Verification items for the finished model (mm, model axes). A direction names the side the tool comes from. Give positions to 0.01 mm unless a question says otherwise; leave off trailing zeros. Loops run counter-clockwise (first coordinate to the right, second up) from the corner with the lowest first, then second, coordinate; pieces in that order, holes last. Notation, with made-up numbers: M 34.5,-26 L 38.5,-26 A18 cw 38.5,2 Z; hole C 77,-32 d4. An arc over 180 degrees is marked long. Use a Markdown table: item, result.
from build123d import *

# Parameters (mm, degrees)
SKETCH_1_W                  = 130
SKETCH_1_H                  = 114
EXTRUDE_1_DEPTH             = 4
CHAMFER_1_SIZE              = 2.5
CHAMFER_1_SIZE2             = 4.330127019
FILLET_1_R                  = 5
FILLET_2_R                  = 3
FILLET_3_R                  = 3
SKETCH_2_R                  = 1.55
CUT_EXTRUDE_1_DEPTH         = 87.544786094
PATTERN_LINEAR_1_COUNT      = 2
PATTERN_LINEAR_1_PITCH      = 116
PATTERN_LINEAR_1_COUNT_DIR2 = 2
PATTERN_LINEAR_1_PITCH_DIR2 = 90
SKETCH_4_R                  = 2.9
CUT_EXTRUDE_2_DEPTH         = 1.8
PATTERN_LINEAR_2_COUNT      = 2
PATTERN_LINEAR_2_PITCH      = 116
PATTERN_LINEAR_2_COUNT_DIR2 = 2
PATTERN_LINEAR_2_PITCH_DIR2 = 90


with BuildPart() as part:
    # Эскиз1 → Бобышка-Вытянуть1 (new body)
    with BuildSketch(Plane(origin=(0, 0, 0), x_dir=(1, 0, 0), z_dir=(0, 1, 0))):
        Rectangle(SKETCH_1_W, SKETCH_1_H)
    extrude(amount=EXTRUDE_1_DEPTH)

    # Фаска1
    chamfer_1_edges = [part.edges().sort_by_distance(p)[0] for p in [
        (0, 4, 57),
    ]]
    chamfer_1_side = [part.faces().sort_by_distance(p)[0] for p in [
        (0, 2, 57),
    ]]
    chamfer(chamfer_1_edges, length=CHAMFER_1_SIZE, length2=CHAMFER_1_SIZE2, reference=chamfer_1_side[0])

    # Скругление1
    fillet_1_edges = [part.edges().sort_by_distance(p)[0] for p in [
        (0, 4, 52.669872981),
    ]]
    fillet(fillet_1_edges, radius=FILLET_1_R)

    # Скругление2
    # the kernel refuses this fillet: 3 mm, written as the material it takes off along each edge
    with BuildSketch(Plane(origin=(69.302949009, 1.5, 57), x_dir=(0, 0.4999999999999978, -0.8660254037844398), z_dir=(-1, 0, 0))) as fillet_2_piece_1:
        with BuildLine():
            CenterArc((1.721179604, 3), FILLET_2_R, 214.540406951, 55.459593049)
            Line((-0.75, 1.299038106), (-0.799423592, 1.265018868))
            ThreePointArc((-0.799423592, 1.265018868), (-0.426961524, 0.619519053), (-0.051961524, -0.03))
            Line((-0.051961524, -0.03), (0, -0.06))
            Line((0, -0.06), (1.721179604, -0.06))
            Line((1.721179604, -0.06), (1.721179604, 0))
        make_face()
    extrude(amount=138.605898019, mode=Mode.SUBTRACT)

    # Скругление3
    fillet_3_edges = [part.edges().sort_by_distance(p)[0] for p in [
        (-65, 2, -57),
        (65, 2, -57),
    ]]
    fillet(fillet_3_edges, radius=FILLET_3_R)

    # Эскиз2 → Вырез-Вытянуть1 (cut, through all)
    with BuildSketch(Plane(origin=(0, 4, 0), x_dir=(1, 0, 0), z_dir=(0, 1, 0))):
        with Locations(Location((-58, 50, 0), (0, 0, 270))):
            Circle(SKETCH_2_R)
    cut_extrude_1 = extrude(amount=-CUT_EXTRUDE_1_DEPTH, mode=Mode.SUBTRACT)

    # Линейный массив1: Cut-Extrude 1 2 × 2
    with Locations(*[(i * PATTERN_LINEAR_1_PITCH, 0, j * PATTERN_LINEAR_1_PITCH_DIR2) for i in range(PATTERN_LINEAR_1_COUNT) for j in range(PATTERN_LINEAR_1_COUNT_DIR2) if (i, j) != (0, 0)]):
        add(cut_extrude_1, mode=Mode.SUBTRACT)

    # Эскиз4 → Вырез-Вытянуть2 (cut)
    with BuildSketch(Plane(origin=(0, 4, 0), x_dir=(1, 0, 0), z_dir=(0, 1, 0))):
        with Locations(Location((-58, 50, 0), (0, 0, 270))):
            Circle(SKETCH_4_R)
    cut_extrude_2 = extrude(amount=-CUT_EXTRUDE_2_DEPTH, mode=Mode.SUBTRACT)

    # Линейный массив2: Cut-Extrude 2 2 × 2
    with Locations(*[(i * PATTERN_LINEAR_2_PITCH, 0, j * PATTERN_LINEAR_2_PITCH_DIR2) for i in range(PATTERN_LINEAR_2_COUNT) for j in range(PATTERN_LINEAR_2_COUNT_DIR2) if (i, j) != (0, 0)]):
        add(cut_extrude_2, mode=Mode.SUBTRACT)


solid = part.part
(1) Cross-section at B-B on z = 40. Record the cut outline in (x, y), then the cut area to 3 significant figures.
Results below:
| item | result |
|---|---|
| outline | M -65,0 L -59.55,0 L -59.55,2.2 L -60.9,2.2 L -60.9,4 L -65,4 Z; M -56.45,0 L 56.45,0 L 56.45,2.2 L 55.1,2.2 L 55.1,4 L -55.1,4 L -55.1,2.2 L -56.45,2.2 Z; M 59.55,0 L 65,0 L 65,4 L 60.9,4 L 60.9,2.2 L 59.55,2.2 Z |
| area | 485 mm^2 |
(2) Draft check along Z on faces 1 (the cylindrical face through (64.1, 2.03, -56.14)), 2 (the cylindrical face through (-60.57, 3.11, -48.66)), 3 (the flat face through (-1, 4, -4)). Enter one of: +Z half, -Z half, draft (parallel to the pull), parting line (faces both ways), or undercut.
Results below:
| item | result |
|---|---|
| face 1 | -Z half |
| face 2 | undercut |
| face 3 | draft |
(3) Gauge pin test, flat ends, axial feed: P1, Ø1, axis at x = -26, y = 2, coming from the +Z side; P2, Ø1.7, axis at x = 59, z = -50, coming from the +Y side; P3, Ø1.9, axis at x = 58, z = 40, coming from the -Y side. Record the tip position at first contact, or that the pin passes through.
Results below:
| item | result |
|---|---|
| P1 | z = 56.46 |
| P2 | y = 2.2 |
| P3 | through |
(4) Cross-section at A-A on x = -58. Record the cut outline in (y, z), then the cut area to 3 significant figures.
Results below:
| item | result |
|---|---|
| outline | M 0,-57 L 4,-57 L 4,-52.9 L 2.2,-52.9 L 2.2,-51.55 L 0,-51.55 Z; M 0,-48.45 L 2.2,-48.45 L 2.2,-47.1 L 4,-47.1 L 4,37.1 L 2.2,37.1 L 2.2,38.45 L 0,38.45 Z; M 0,41.55 L 2.2,41.55 L 2.2,42.9 L 4,42.9 L 4,51.33 A5 ccw 3.33,53.83 L 2.36,55.51 A3 ccw 0,57 Z |
| area | 415 mm^2 |
(5) Set-up check for faces 4 (the flat face through (56.75, 2.2, -48.75)), 5 (the cylindrical face through (-57.534, 1.115, -48.522)): record each of +Z, -Z, +X, -X, +Y, -Y from which the full face is reachable in a straight line by a thin tool's end or side.
Results below:
| item | result |
|---|---|
| face 4 | +Y |
| face 5 | +Y, -Y |
(6) Material ranges on line 1 (X direction, y = 3.55, z = -50); line 2 (X direction, y = 0.75, z = -50); line 3 (Z direction, x = 41, y = 0.2), recorded low to high.
Results below:
| item | result |
|---|---|
| line 1 | -65 to -60.9, -55.1 to 55.1, 60.9 to 65 |
| line 2 | -65 to -59.55, -56.45 to 56.45, 59.55 to 65 |
| line 3 | -57 to 56.98 |
